from build123d import *

# Parameters (mm, degrees)
SKETCH1_R           = 1.5
SKETCH1_R_2         = 2
BOSS_EXTRUDE1_DEPTH = 6.35
FILLET1_R           = 2
SKETCH2_R           = 2.1
BOSS_EXTRUDE2_DEPTH = 6.35


with BuildPart() as part:
    # Sketch1 → Boss-Extrude1 (new body)
    with BuildSketch(Plane.XY):
        with BuildLine():
            Line((25.95, 45.499996), (25.95, 9.999996))
            Line((25.95, 9.999996), (34.9, 9.999996))
            Line((34.9, 9.999996), (34.9, -10))
            Line((34.9, -10), (5, -10))
            Line((5, -10), (5, 9.999996))
            Line((5, 9.999996), (13.95, 9.999996))
            Line((13.95, 9.999996), (13.95, 45.499996))
            ThreePointArc((13.95, 45.499996), (19.95, 51.499996), (25.95, 45.499996))
        make_face()
        with Locations((27.95, -7.5)):
            Circle(SKETCH1_R, mode=Mode.SUBTRACT)
        with Locations((11.95, -7.5)):
            Circle(SKETCH1_R, mode=Mode.SUBTRACT)
        with Locations((27.95, 7.5)):
            Circle(SKETCH1_R, mode=Mode.SUBTRACT)
        with Locations((11.95, 7.5)):
            Circle(SKETCH1_R, mode=Mode.SUBTRACT)
        with Locations((19.95, 45.499996)):
            Circle(SKETCH1_R_2, mode=Mode.SUBTRACT)
        with Locations((19.95, 20.499996)):
            Circle(SKETCH1_R_2, mode=Mode.SUBTRACT)
    extrude(amount=BOSS_EXTRUDE1_DEPTH)

    # Fillet1
    fillet1_edges = [part.edges().sort_by_distance(p)[0] for p in [
        (5, 9.999996, 3.175),
        (13.95, 9.999996, 3.175),
        (25.95, 9.999996, 3.175),
        (34.9, 9.999996, 3.175),
        (34.9, -10, 3.175),
        (5, -10, 3.175),
    ]]
    fillet(fillet1_edges, radius=FILLET1_R)

    # Sketch2 → Boss-Extrude2 (add)
    with BuildSketch(Plane.XY.offset(6.35)):
        with BuildLine():
            Line((24.559539107, 49.340848668), (39.791282589, 31.060710557))
            ThreePointArc((39.791282589, 31.060710557), (40.778341906, 29.158889693), (40.87868421, 27.018529882))
            Line((40.87868421, 27.018529882), (34.9, -8))
            Line((34.9, -8), (34.9, 7.999996))
            ThreePointArc((34.9, 7.999996), (34.314213562, 9.414209562), (32.9, 9.999996))
            Line((32.9, 9.999996), (27.95, 9.999996))
            ThreePointArc((27.95, 9.999996), (26.535786438, 10.585782437), (25.95, 11.999996))
            Line((25.95, 11.999996), (25.95, 45.499996))
            ThreePointArc((25.95, 45.499996), (25.591685681, 47.542392308), (24.559539107, 49.340848668))
        make_face()
        with Locations((35.95, 27.86)):
            Circle(SKETCH2_R, mode=Mode.SUBTRACT)
    extrude(amount=-BOSS_EXTRUDE2_DEPTH)


solid = part.part
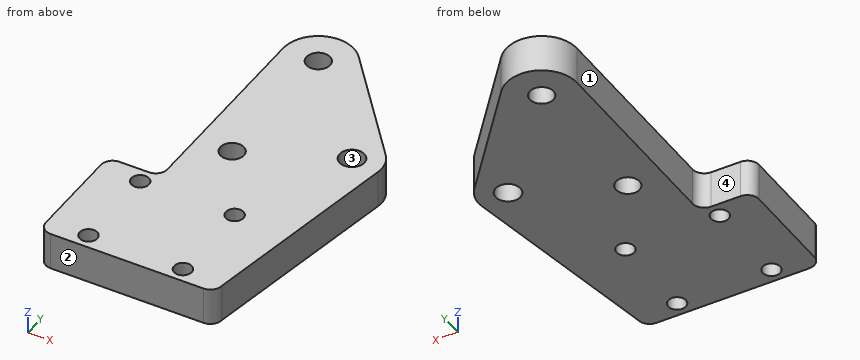
For this review, take the finished solid that the model builds, in its own axes (mm). Face numbers are marked on the shaded views. Round coordinates to 2 decimals unless told otherwise and drop trailing zeros. Order: outer loops, then holes, each group sorted by start corner. A loop starts at its lowest first (then second) coordinate and runs counter-clockwise, first axis right, second up. Notation, with made-up numbers: M 67,71.25 L 91,71.25 A19 ccw 91,79.25 Z; hole C -28.5,73.25 d6. An arc over 180 degrees is marked long. Use a Markdown table: item, result. Add a question column.
Item 1: Add section B-B, the plane x = 19.95. Give the boundary of the cut face in (y, z), then the cut area to 3 significant figures.
Item 2: To check wall thickness, follow line 1 along Y through (x, z) = (19.95, 2.5); line 2 along Y through (x, z) = (27.95, 2.5); line 3 along X through (y, z) = (31, 5.75). State the ranges of each line that lie inside material, in increasing order.
Item 3: Add section C-C, the plane x = 35.95. Give the boundary of the cut face in (y, z), then the cut area to 3 significant figures.
Item 4: Insertion check: pin 1 (4 mm diameter, centred on x = 27.95, y = -7.5, fed in from +Z); pin 2 (3 mm diameter, centred on y = 25, z = 2, fed in from -X); pin 3 (1 mm diameter, centred on y = -2.5, z = 5, fed in from +X); pin 4 (2.5 mm diameter, centred on x = 9, z = 2.5, fed in from +Y). Each pin has a flat end and moves straight along its axis. Give the tip position at first contact, or say it passes through.
Item 5: Add section D-D, the plane z = 2. Give the boundary of the cut face in (x, y).
Item 6: Add section A-A, the plane y = 27.86. Give the boundary of the cut face in (x, z).
Item 7: Mouldability with a two-part tool opening along Y and no side actions: class the marked faces 1, 2, 3 and 4 as released by +Y, released by -Y, zero draft, split by the parting line, or undercut.
Geometry results:
| question | item | result |
|---|---|---|
| 1 | outline | M -10,0 L 18.5,0 L 18.5,6.35 L -10,6.35 Z; M 22.5,0 L 43.5,0 L 43.5,6.35 L 22.5,6.35 Z; M 47.5,0 L 51.5,0 L 51.5,6.35 L 47.5,6.35 Z |
| 1 | area | 340 mm² |
| 2 | line 1 | y = -10 to 18.5, 22.5 to 43.5, 47.5 to 51.5 |
| 2 | line 2 | y = -10 to -9, -6 to 6, 9 to 45.27 |
| 2 | line 3 | x = 13.95 to 39.84 |
| 3 | outline | M -1.85,0 L 25.76,0 L 25.76,6.35 L -1.85,6.35 Z; M 29.96,0 L 35.67,0 L 35.67,6.35 L 29.96,6.35 Z |
| 3 | area | 212 mm² |
| 4 | pin 1 | stops at z = 6.35 |
| 4 | pin 2 | stops at x = 13.95 |
| 4 | pin 3 | stops at x = 35.92 |
| 4 | pin 4 | stops at y = 10 |
| 5 | outline | M 5,-8 A2 ccw 7,-10 L 32.9,-10 A2 ccw 34.9,-8 L 40.88,27.02 A5 ccw 39.79,31.06 L 24.56,49.34 A6 ccw 13.95,45.5 L 13.95,12 A2 cw 11.95,10 L 7,10 A2 ccw 5,8 Z; hole C 11.95,-7.5 d3; hole C 11.95,7.5 d3; hole C 19.95,20.5 d4; hole C 19.95,45.5 d4; hole C 27.95,-7.5 d3; hole C 27.95,7.5 d3; hole C 35.95,27.86 d4.2 |
| 6 | outline | M 13.95,0 L 33.85,0 L 33.85,6.35 L 13.95,6.35 Z; M 38.05,0 L 40.95,0 L 40.95,6.35 L 38.05,6.35 Z |
| 7 | face 1 | zero draft |
| 7 | face 2 | released by -Y |
| 7 | face 3 | undercut |
| 7 | face 4 | released by +Y |
